Could you check a few things on this model? Use its own coordinates, in mm. A direction names the side the tool comes from. Round coordinates to 2 decimals unless told otherwise and drop trailing zeros. Loops run counter-clockwise (first coordinate to the right, second up) from the corner with the lowest first, then second, coordinate; pieces in that order, holes last. Notation, with made-up numbers: (9.5, 5) -> (59.5, 5) arc R22 ccw to (59.5, 34) -> close; hole circle Ø10 at (84, 67). An arc over 180 degrees is marked (long way). Put each result on its own line as item: value. Start each with the question number.
1. Imagine slicing it at B-B, the plane z = 48.5. Please give me the cut outline in (x, y).
2. I need wall thicknesses on line 1 (X direction, y = -1.4, z = 114.5); line 2 (Z direction, x = 2.25, y = -14.25); line 3 (Y direction, x = -4.5, z = 61). Which ranges of each line are inside material? Lowest first, please. Write a range as [from, to].
3. Which directions (+Z, -Z, +X, -X, +Y, -Y) give clear straight access to the entire face, cutting with the end or side of a thin tool? Please do faces 5 (the flat face through (0, -13, 25)), 6 (the flat face through (0, -10, 0)), 7 (the flat face through (5, -5, 54)), 8 (the flat face through (0, -19.5, 10)), 9 (the flat face through (-5, -5, 55)).
4. Imagine slicing it at A-A, the plane y = -4.25. Please give me the cut outline in (x, z).
5. I'm going to push flat-ended pins straight in: P1, Ø3, axis at x = -1.5, z = 89, coming from the -Y side; P2, Ø2, axis at y = -7, z = 14.5, coming from the -X side; P3, Ø10, axis at y = -10.5, z = 84.5, coming from the -X side; P4, Ø2.5, axis at x = 0, z = 114.5, coming from the -Y side. Where does each tip first touch, or does it pass through?
6. If we mould it in two halves opening along Z, with no side actions, what happens to faces 1 (the cylindrical face through (0, -3, 47)), 2 (the flat face through (0, -3, 120)), 3 (the cylindrical face through (0, -3, 116)), 4 (the flat face through (0, -6, 73))? For each: pulls with the +Z half, pulls with the -Z half, needs draft (parallel to the pull), parting line crosses it, or undercut.
7. Imagine slicing it at D-D, the plane x = 3.5. Please give me the cut outline in (y, z), and give its area (3 significant figures).
8. Imagine slicing it at C-C, the plane y = -9.25. Please give me the cut outline in (x, z).
```python
from build123d import *

# Parameters (mm, degrees)
F1_DEPTH = 19.5
F0_R     = 1.5
F2_DEPTH = 6
F3_R     = 3


with BuildPart() as f1:
    # F0 (on Front) → F1 (new body)
    with BuildSketch(Plane.XZ):
        with BuildLine():
            Line((-9, 0), (0, 0))
            Line((0, 0), (0, 6))
            ThreePointArc((0, 6), (-1.5, 7.5), (0, 9))
            Line((0, 9), (0, 25))
            Line((0, 25), (-5, 25))
            Line((-5, 25), (-5, 15))
            Line((-5, 15), (-9, 0))
        make_face()
        with BuildLine():
            Line((0, 6), (0, 0))
            Line((0, 0), (9, 0))
            Line((9, 0), (5, 15))
            Line((5, 15), (5, 25))
            Line((5, 25), (0, 25))
            Line((0, 25), (0, 9))
            ThreePointArc((0, 9), (1.06066, 8.56066), (1.5, 7.5))
            ThreePointArc((1.5, 7.5), (1.06066, 6.43934), (0, 6))
        make_face()
    extrude(amount=F1_DEPTH)

    # F0 (on Front) → F2 (join)
    with BuildSketch(Plane.XZ):
        Polygon((0, 25), (5, 25), (5, 120), (-5, 120), (-5, 25), align=None)
        with Locations((0, 48.5)):
            Circle(F0_R, mode=Mode.SUBTRACT)
        with Locations((0, 114.5)):
            Circle(F0_R, mode=Mode.SUBTRACT)
    extrude(amount=F2_DEPTH)

    # F3
    f3_edges = [f1.edges().sort_by_distance(p)[0] for p in [
        (5, -3, 120),
        (-5, -3, 120),
        (9, -9.75, 0),
        (-9, -9.75, 0),
    ]]
    fillet(f3_edges, radius=F3_R)


solid = f1.part
```
Entries:
1. outline: (-5, -6) -> (-1.5, -6) -> (-1.5, 0) -> (-5, 0) -> close; (1.5, -6) -> (5, -6) -> (5, 0) -> (1.5, 0) -> close
2. line 1: [-5, -1.5], [1.5, 5]
2. line 2: [0, 25]
2. line 3: [-6, 0]
3. face 5: +Z, +X, -X, -Y
3. face 6: -Z, +X, -X, +Y, -Y
3. face 7: +Z, +X, +Y, -Y
3. face 8: +Z, -Z, +X, -X, -Y
3. face 9: +Z, -X, +Y, -Y
4. outline: (-7.99, 3.77) arc R3 ccw to (-5.1, 0) -> (5.1, 0) arc R3 ccw to (7.99, 3.77) -> (5, 15) -> (5, 117) arc R3 ccw to (2, 120) -> (-2, 120) arc R3 ccw to (-5, 117) -> (-5, 15) -> close; hole circle Ø3 at (0, 7.5); hole circle Ø3 at (0, 48.5); hole circle Ø3 at (0, 114.5)
5. P1: y = -6
5. P2: x = -5.4
5. P3: x = -5
5. P4: through
6. face 1: undercut
6. face 2: pulls with the +Z half
6. face 3: undercut
6. face 4: needs draft
7. outline: (-19.5, 0) -> (0, 0) -> (0, 119.6) -> (-6, 119.6) -> (-6, 25) -> (-19.5, 25) -> close
7. area: 1,060 mm^2
8. outline: (-7.99, 3.77) arc R3 ccw to (-5.1, 0) -> (5.1, 0) arc R3 ccw to (7.99, 3.77) -> (5, 15) -> (5, 25) -> (-5, 25) -> (-5, 15) -> close; hole circle Ø3 at (0, 7.5)
